```python
from build123d import *

# Parameters (mm, degrees)
SKETCH1_R           = 1.7145
SKETCH1_W           = 0.79375
SKETCH1_H           = 19.05
SKETCH1_R_2         = 1.5875
BOSS_EXTRUDE1_DEPTH = 3.175


with BuildPart() as part:
    # Sketch1 → Boss-Extrude1 (new body)
    with BuildSketch(Plane.XY.offset(-196.85)):
        with BuildLine():
            Line((-85.725, -136.525), (-94.488, -136.525))
            Line((-94.488, -136.525), (-94.488, -171.45))
            ThreePointArc((-94.488, -171.45), (-91.334797487, -183.509623583), (-82.682291667, -192.482435298))
            ThreePointArc((-82.682291667, -192.482435298), (-76.266849592, -192.599023491), (-73.025, -187.061704551))
            Line((-73.025, -187.061704551), (-73.025, -153.666835653))
            ThreePointArc((-73.025, -153.666835653), (-72.058270063, -148.806756062), (-69.305256121, -144.686579532))
            Line((-69.305256121, -144.686579532), (-52.819423728, -128.200747139))
            ThreePointArc((-52.819423728, -128.200747139), (-48.699247198, -125.447733197), (-43.839167607, -124.48100326))
            Line((-43.839167607, -124.48100326), (43.839167607, -124.48100326))
            ThreePointArc((43.839167607, -124.48100326), (48.699247198, -125.447733197), (52.819423728, -128.200747139))
            Line((52.819423728, -128.200747139), (69.305256121, -144.686579532))
            ThreePointArc((69.305256121, -144.686579532), (72.058270063, -148.806756062), (73.025, -153.666835653))
            Line((73.025, -153.666835653), (73.025, -187.061704551))
            ThreePointArc((73.025, -187.061704551), (76.266849592, -192.599023491), (82.682291667, -192.482435298))
            ThreePointArc((82.682291667, -192.482435298), (91.334797487, -183.509623583), (94.488, -171.45))
            Line((94.488, -171.45), (94.488, -136.525))
            Line((94.488, -136.525), (85.725, -136.525))
            Line((85.725, -136.525), (85.725, -115.57))
            ThreePointArc((85.725, -115.57), (85.353025612, -114.671974388), (84.455, -114.3))
            Line((84.455, -114.3), (63.5, -114.3))
            Line((63.5, -114.3), (63.5, -111.125))
            Line((63.5, -111.125), (94.488, -111.125))
            Line((94.488, -111.125), (94.488, -85.725))
            Line((94.488, -85.725), (88.9, -85.725))
            Line((88.9, -85.725), (88.9, -60.325))
            Line((88.9, -60.325), (94.488, -60.325))
            Line((94.488, -60.325), (94.488, -25.4))
            ThreePointArc((94.488, -25.4), (87.271696875, -7.978303125), (69.85, -0.762))
            Line((69.85, -0.762), (-69.85, -0.762))
            ThreePointArc((-69.85, -0.762), (-87.271696875, -7.978303125), (-94.488, -25.4))
            Line((-94.488, -25.4), (-94.488, -60.325))
            Line((-94.488, -60.325), (-88.9, -60.325))
            Line((-88.9, -60.325), (-88.9, -85.725))
            Line((-88.9, -85.725), (-94.488, -85.725))
            Line((-94.488, -85.725), (-94.488, -111.125))
            Line((-94.488, -111.125), (-63.5, -111.125))
            Line((-63.5, -111.125), (-63.5, -114.3))
            Line((-63.5, -114.3), (-84.455, -114.3))
            ThreePointArc((-84.455, -114.3), (-85.353025612, -114.671974388), (-85.725, -115.57))
            Line((-85.725, -115.57), (-85.725, -136.525))
        make_face()
        with Locations((-79.375, -180.213)):
            Circle(SKETCH1_R, mode=Mode.SUBTRACT)
        with Locations((-89.296875, -158.75)):
            Rectangle(SKETCH1_W, SKETCH1_H, mode=Mode.SUBTRACT)
        with Locations((-38.1, -111.125)):
            Circle(SKETCH1_R, mode=Mode.SUBTRACT)
        with Locations((79.375, -180.213)):
            Circle(SKETCH1_R, mode=Mode.SUBTRACT)
        with Locations((89.296875, -158.75)):
            Rectangle(SKETCH1_W, SKETCH1_H, mode=Mode.SUBTRACT)
        with Locations((38.1, -111.125)):
            Circle(SKETCH1_R, mode=Mode.SUBTRACT)
        with BuildLine():
            ThreePointArc((-67.060192091, -72.204012806), (-69.124952547, -69.113880409), (-69.85, -65.468820715))
            Line((-69.85, -65.468820715), (-69.85, -40.839204897))
            ThreePointArc((-69.85, -40.839204897), (-66.714031836, -36.145896872), (-61.177897552, -37.247102448))
            Line((-61.177897552, -37.247102448), (-18.197102448, -80.227897552))
            ThreePointArc((-18.197102448, -80.227897552), (-17.095896872, -85.764031836), (-21.789204897, -88.9))
            Line((-21.789204897, -88.9), (-46.418820715, -88.9))
            ThreePointArc((-46.418820715, -88.9), (-50.063880409, -88.174952547), (-53.154012806, -86.110192091))
            Line((-53.154012806, -86.110192091), (-67.060192091, -72.204012806))
        make_face(mode=Mode.SUBTRACT)
        with Locations((-69.85, -25.4)):
            Circle(SKETCH1_R_2, mode=Mode.SUBTRACT)
        with Locations((-19.05, -12.7)):
            Circle(SKETCH1_R_2, mode=Mode.SUBTRACT)
        with BuildLine():
            ThreePointArc((3.592102448, -81.36251337), (0, -82.850410922), (-3.592102448, -81.36251337))
            Line((-3.592102448, -81.36251337), (-50.88251337, -34.072102448))
            ThreePointArc((-50.88251337, -34.072102448), (-51.983718947, -28.535968164), (-47.290410922, -25.4))
            Line((-47.290410922, -25.4), (47.290410922, -25.4))
            ThreePointArc((47.290410922, -25.4), (51.983718947, -28.535968164), (50.88251337, -34.072102448))
            Line((50.88251337, -34.072102448), (3.592102448, -81.36251337))
        make_face(mode=Mode.SUBTRACT)
        with BuildLine():
            ThreePointArc((53.154012806, -86.110192091), (50.063880409, -88.174952547), (46.418820715, -88.9))
            Line((46.418820715, -88.9), (21.789204897, -88.9))
            ThreePointArc((21.789204897, -88.9), (17.095896872, -85.764031836), (18.197102448, -80.227897552))
            Line((18.197102448, -80.227897552), (61.177897552, -37.247102448))
            ThreePointArc((61.177897552, -37.247102448), (66.714031836, -36.145896872), (69.85, -40.839204897))
            Line((69.85, -40.839204897), (69.85, -65.468820715))
            ThreePointArc((69.85, -65.468820715), (69.124952547, -69.113880409), (67.060192091, -72.204012806))
            Line((67.060192091, -72.204012806), (53.154012806, -86.110192091))
        make_face(mode=Mode.SUBTRACT)
        with Locations((19.05, -12.7)):
            Circle(SKETCH1_R_2, mode=Mode.SUBTRACT)
        with Locations((69.85, -25.4)):
            Circle(SKETCH1_R_2, mode=Mode.SUBTRACT)
    extrude(amount=-BOSS_EXTRUDE1_DEPTH)


solid = part.part
```
Part model, mm, in its own coordinate system. A direction names the side the tool comes from. Give positions to 0.01 mm unless a question says otherwise; leave off trailing zeros. Write each loop counter-clockwise with the first axis right and the second up, starting at its lowest first coordinate (ties: lowest second). Pieces come first, ordered by that corner, then holes. Notation, with made-up numbers: M 21,85.5 L 58,85.5 A14 ccw 58,96.5 Z; hole C -16.75,38 d3. An arc over 180 degrees is marked long. Use CSV: the item, a comma, the result in double quotes.
Item 1: Which spindle directions (+Z, -Z, +X, -X, +Y, -Y) get a long thin tool onto all of the face, cutting with end or side? Do faces 4 (the face through (27.568, -57.386, -198.415)), 5 (the face through (-61.18, -136.56, -198.42)), 6 (the face through (-91.42, -183.36, -198.42)). Say none if no direction does.
Taken from the geometry:
face 4,"+Z, -Z"
face 5,"+Z, -Z, -Y"
face 6,"+Z, -Z, -X, -Y"
Item 2: Pull direction X, two halves, no side cores. Call faces 1 (the face through (-76.349, -192.645, -198.415)), 2 (the face through (-1, -96, -196.85)), 3 (the face through (87.46, -8.17, -198.42)): +X half, -X half, draft (parallel to the pull), parting line (faces both ways), or undercut.
Taken from the geometry:
face 1,"undercut"
face 2,"draft"
face 3,"+X half"
Item 3: Slice it at B-B on x = -58. Write the cut outline in (y, z) (3 decimals), plus the area to 3 significant figures.
Taken from the geometry:
outline,"M -133.381,-200.025 L -81.264,-200.025 L -81.264,-196.85 L -133.381,-196.85 Z; M -40.425,-200.025 L -0.762,-200.025 L -0.762,-196.85 L -40.425,-196.85 Z"
area,"291 mm²"
Item 4: Pin check, flat tips, straight feed: P1, Ø1.6, axis at y = -131, z = -199, coming from the -X side (3 decimals); P2, Ø0.9, axis at x = 89.5, z = -198, coming from the +Y side; P3, Ø1, axis at x = 75.5, z = -198, coming from the -Y side. Stop position of each tip, or through.
Taken from the geometry:
P1,"stops at x = -85.725"
P2,"stops at y = -9.96"
P3,"stops at y = -192.44"
Item 5: Slice it at A-A on y = -63. Write the cut outline in (x, z) (3 decimals), plus the area to 3 significant figures.
Taken from the geometry:
outline,"M -88.9,-200.025 L -69.85,-200.025 L -69.85,-196.85 L -88.9,-196.85 Z; M -35.425,-200.025 L -21.955,-200.025 L -21.955,-196.85 L -35.425,-196.85 Z; M 21.955,-200.025 L 35.425,-200.025 L 35.425,-196.85 L 21.955,-196.85 Z; M 69.85,-200.025 L 88.9,-200.025 L 88.9,-196.85 L 69.85,-196.85 Z"
area,"207 mm²"
Item 6: Slice it at C-C on z = -197.55. State how many separate pieces and enclosed holes the cut face has, plus the area to 3 significant figures.
Taken from the geometry:
separate pieces,"1"
enclosed holes,"13"
area,"18,900 mm²"
Item 7: Drill centre lines: probe 1 along X at (y, z) = (-152.5, -197.8); probe 2 along Y at (x, z) = (38.1, -198.7) (1 decimal); probe 3 along X at (y, z) = (-86, -199.05). Where is each one in solid material? Low to high.
Taken from the geometry:
probe 1,"x = -94.49 to -89.69, -88.9 to -72.97, 72.97 to 88.9, 89.69 to 94.49"
probe 2,"y = -124.5 to -112.8, -109.4 to -88.9, -60.3 to -46.9, -25.4 to -0.8"
probe 3,"x = -94.49 to -53.26, -17.2 to 17.2, 53.26 to 94.49"
